Geometry: see drawing. Coordinates: mm, zero at the bounding-box minimum. A direction names the side the tool comes from. Round coordinates to 2 decimals unless told otherwise and drop trailing zeros. Loops run counter-clockwise (first coordinate to the right, second up) from the corner with the lowest first, then second, coordinate; pieces in that order, holes last.
(1) Section C-C, the plane x = 14.5. Return the cut outline in (y, z), plus the area to 3 significant figures.
(2) Section B-B, the plane y = 16. Return the cut outline in (x, z).
(3) Set-up query: the marked faces 1 and 2. Return all of +Z, -Z, +X, -X, +Y, -Y with unobstructed straight access to the full face (end or side cutting, diameter ignored); none if empty.
(4) Section A-A, the plane z = 0.9. Return the cut outline in (x, y), plus the area to 3 significant figures.
(5) First-contact query: pin 1 Ø1.2 at (y, z) = (14.5, 1) entering from -X; pin 2 Ø1.5 at (x, z) = (30, 1) entering from +Y; pin 3 Ø8 at (x, y) = (13.5, 27) entering from -Z; pin 4 Ø2 at (x, z) = (4, 1.5) entering from -Y. Flat tips, straight axial feed; report the tip coordinate or a pass-through.
(6) Material intervals for probe 1 along X at (y, z) = (22, 0.7); probe 2 along Y at (x, z) = (5, 1.3); probe 3 along Y at (x, z) = (28.5, 1.35), sorted ascending.
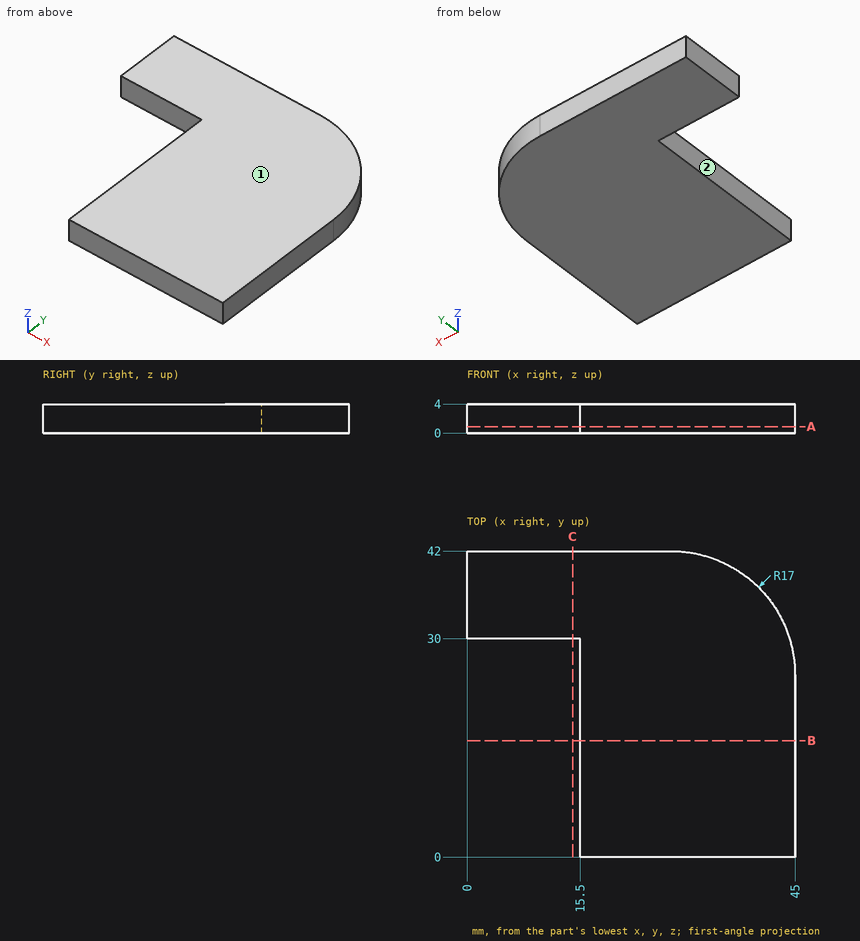
Output values:
1. outline: (30, 0) - (42, 0) - (42, 4) - (30, 4) - close
1. area: 48.0 mm2
2. outline: (15.5, 0) - (45, 0) - (45, 4) - (15.5, 4) - close
3. face 1: +Z, +X, -X, +Y, -Y
3. face 2: +Z, -Z, -X, -Y
4. outline: (0, 30) - (15.5, 30) - (15.5, 0) - (45, 0) - (45, 25) arc R17 ccw to (28, 42) - (0, 42) - close
4. area: 1,360 mm2
5. pin 1: stops at x = 15.5
5. pin 2: stops at y = 41.95
5. pin 3: stops at z = 0
5. pin 4: stops at y = 30
6. probe 1: x = 15.5 to 45
6. probe 2: y = 30 to 42
6. probe 3: y = 0 to 41.99
